Can you work these out from the model? Positions are in its coordinate system, mm. Face numbers are marked on the shaded views. Give positions to 0.01 mm unless a question says otherwise; leave off trailing zeros. Order: outer loops, then holes, each group sorted by start corner. A loop starts at its lowest first (then second) coordinate and runs counter-clockwise, first axis right, second up. Notation, with made-up numbers: (70.25, -39.5) -> (85.25, -39.5) arc R20 ccw to (85.25, -14.5) -> close; hole circle Ø4 at (-2, 41). An arc over 180 degrees is marked (long way). Answer as a JSON object with one key per item and string values.
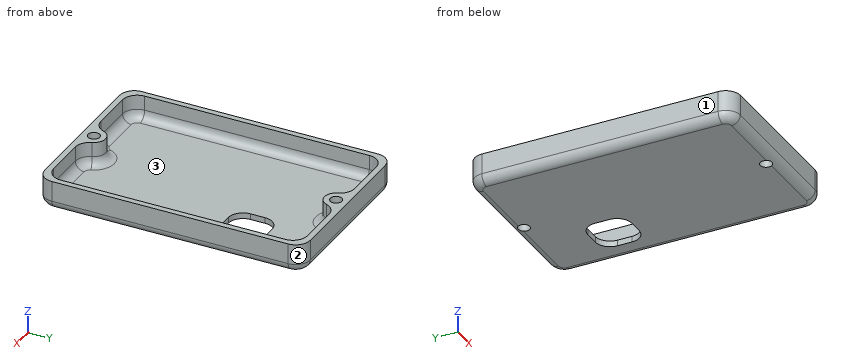
```python
from build123d import *

# Parameters (mm, degrees)
F3_W          = 60
F3_H          = 91
F4_DEPTH      = 10
F5_W          = 56
F5_H          = 87
F6_DEPTH      = 8
F7_R          = 4
F8_DEPTH      = 10
F9_R          = 2
F10_DEPTH     = 10.001
F11_R         = 5
F12_R         = 5
F13_T1_DEPTH  = 77
F13_T3_DEPTH  = 14.5147186258
F13_T5_DEPTH  = 14.5147186258
F13_T8_ANGLE  = 90
F13_T10_ANGLE = 70.5287793655
F13_T12_ANGLE = 141.057558731
F13_T14_ANGLE = 90
F13_T16_ANGLE = 70.5287793655
F13_T18_ANGLE = 70.5287793655
F13_T20_ANGLE = 90
F13_T22_ANGLE = 141.057558731
F13_T24_ANGLE = 70.5287793655
F13_T26_ANGLE = 90
F13_T27_DEPTH = 81
F13_T29_DEPTH = 50
F13_T32_ANGLE = 90
F13_T34_ANGLE = 90
F13_T36_ANGLE = 90
F13_T38_ANGLE = 90
F14_W         = 15
F14_H         = 15
F15_DEPTH     = 2.0010001
F16_R         = 5


# Not quite as in the source:
# - a fillet or chamfer that OpenCascade refuses, or shapes differently, is made with other operations: its cross-section is extruded or revolved along the edge and cut away or added


with BuildPart() as f4:
    # F3 (on Top) → F4 (new body)
    with BuildSketch(Plane.XY):
        Rectangle(F3_W, F3_H)
    extrude(amount=F4_DEPTH)

    # F5 (on face) → F6 (cut)
    with BuildSketch(Plane.XY.offset(10)):
        Rectangle(F5_W, F5_H)
    extrude(amount=-F6_DEPTH, mode=Mode.SUBTRACT)

    # F7 (on face) → F8 (join)
    with BuildSketch(Plane(origin=(0, 0, 0), x_dir=(1, 0, 0), z_dir=(0, 0, -1))):
        with Locations((0, -41.5)):
            Circle(F7_R)
        with Locations((0, 41.5)):
            Circle(F7_R)
    extrude(amount=-F8_DEPTH)

    # F9 (on face) → F10 (cut, through all)
    with BuildSketch(Plane(origin=(0, 0, 0), x_dir=(1, 0, 0), z_dir=(0, 0, -1))):
        with Locations((0, -41.5)):
            Circle(F9_R)
        with Locations((0, 41.5)):
            Circle(F9_R)
    extrude(amount=-F10_DEPTH, mode=Mode.SUBTRACT)

    # F11
    f11_edges = [f4.edges().sort_by_distance(p)[0] for p in [
        (3.464102, 43.5, 6),
        (-3.464102, 43.5, 6),
        (-3.464102, -43.5, 6),
        (3.464102, -43.5, 6),
    ]]
    fillet(f11_edges, radius=F11_R)

    # F12
    f12_edges = [f4.edges().sort_by_distance(p)[0] for p in [
        (30, -45.5, 5),
        (-30, -45.5, 5),
        (30, 45.5, 5),
        (-30, 45.5, 5),
        (28, -43.5, 6),
        (-28, -43.5, 6),
        (-28, 43.5, 6),
        (28, 43.5, 6),
    ]]
    fillet(f12_edges, radius=F12_R)

    # F13: fillet of radius 3 on 24 edges, made by hand

    # F13_s2 → F13_t1 (join)
    with BuildSketch(Plane.XZ.offset(-38.5)):
        with BuildLine():
            ThreePointArc((-28, 5), (-27.1213203436, 2.8786796564), (-25, 2))
            Line((-25, 2), (-28, 2))
            Line((-28, 2), (-28, 5))
        make_face()
        with BuildLine():
            ThreePointArc((28, 5), (27.1213203436, 2.8786796564), (25, 2))
            Line((25, 2), (28, 2))
            Line((28, 2), (28, 5))
        make_face()
    extrude(amount=F13_T1_DEPTH)

    # F13_s4 → F13_t3 (join)
    with BuildSketch(Plane.YZ.offset(8.4852813742)):
        with BuildLine():
            ThreePointArc((-43.5, 5), (-42.6213203436, 2.8786796564), (-40.5, 2))
            Line((-40.5, 2), (-43.5, 2))
            Line((-43.5, 2), (-43.5, 5))
        make_face()
        with BuildLine():
            ThreePointArc((43.5, 5), (42.6213203436, 2.8786796564), (40.5, 2))
            Line((40.5, 2), (43.5, 2))
            Line((43.5, 2), (43.5, 5))
        make_face()
    extrude(amount=F13_T3_DEPTH)

    # F13_s6 → F13_t5 (join)
    with BuildSketch(Plane.YZ.offset(-23)):
        with BuildLine():
            ThreePointArc((-43.5, 5), (-42.6213203436, 2.8786796564), (-40.5, 2))
            Line((-40.5, 2), (-43.5, 2))
            Line((-43.5, 2), (-43.5, 5))
        make_face()
        with BuildLine():
            ThreePointArc((43.5, 5), (42.6213203436, 2.8786796564), (40.5, 2))
            Line((40.5, 2), (43.5, 2))
            Line((43.5, 2), (43.5, 5))
        make_face()
    extrude(amount=F13_T5_DEPTH)

    # F13_s7 → F13_t8 (revolve)
    with BuildSketch(Plane.YZ.offset(23)):
        with BuildLine():
            ThreePointArc((-43.5, 5), (-42.6213203436, 2.8786796564), (-40.5, 2))
            Line((-40.5, 2), (-43.5, 2))
            Line((-43.5, 2), (-43.5, 5))
        make_face()
    revolve(axis=Axis((23, -38.5, 2), (0, 0, 1)), revolution_arc=F13_T8_ANGLE)

    # F13_s9 → F13_t10 (revolve)
    with BuildSketch(Plane.YZ.offset(8.4852813742)):
        with BuildLine():
            ThreePointArc((-43.5, 5), (-42.6213203436, 2.8786796564), (-40.5, 2))
            Line((-40.5, 2), (-43.5, 2))
            Line((-43.5, 2), (-43.5, 5))
        make_face()
    revolve(axis=Axis((8.4852813742, -38.5, 2), (0, 0, -1)), revolution_arc=F13_T10_ANGLE)

    # F13_s11 → F13_t12 (revolve)
    with BuildSketch(Plane(origin=(-13.0421917419, -36.8888888889, 0), x_dir=(0, 0, 1), z_dir=(-0.3333333333, -0.9428090416, 0))):
        with BuildLine():
            ThreePointArc((5, -9.8333333333), (2.8786796564, -8.9546536769), (2, -6.8333333333))
            Line((2, -6.8333333333), (2, -9.8333333333))
            Line((2, -9.8333333333), (5, -9.8333333333))
        make_face()
    revolve(axis=Axis((0, -41.5, 2), (0, 0, -1)), revolution_arc=F13_T12_ANGLE)

    # F13_s13 → F13_t14 (revolve)
    with BuildSketch(Plane.XZ.offset(-38.5)):
        with BuildLine():
            ThreePointArc((28, 5), (27.1213203436, 2.8786796564), (25, 2))
            Line((25, 2), (28, 2))
            Line((28, 2), (28, 5))
        make_face()
    revolve(axis=Axis((23, 38.5, 2), (0, 0, 1)), revolution_arc=F13_T14_ANGLE)

    # F13_s15 → F13_t16 (revolve)
    with BuildSketch(Plane(origin=(-13.0421917419, -36.8888888889, 0), x_dir=(0, 0, 1), z_dir=(0.3333333333, 0.9428090416, 0))):
        with BuildLine():
            ThreePointArc((5, 9.8333333333), (2.8786796564, 8.9546536769), (2, 6.8333333333))
            Line((2, 6.8333333333), (2, 9.8333333333))
            Line((2, 9.8333333333), (5, 9.8333333333))
        make_face()
    revolve(axis=Axis((-8.4852813742, -38.5, 2), (0, 0, -1)), revolution_arc=F13_T16_ANGLE)

    # F13_s17 → F13_t18 (revolve)
    with BuildSketch(Plane.YZ.offset(8.4852813742)):
        with BuildLine():
            ThreePointArc((43.5, 5), (42.6213203436, 2.8786796564), (40.5, 2))
            Line((40.5, 2), (43.5, 2))
            Line((43.5, 2), (43.5, 5))
        make_face()
    revolve(axis=Axis((8.4852813742, 38.5, 2), (0, 0, 1)), revolution_arc=F13_T18_ANGLE)

    # F13_s19 → F13_t20 (revolve)
    with BuildSketch(Plane.YZ.offset(-23)):
        with BuildLine():
            ThreePointArc((-43.5, 5), (-42.6213203436, 2.8786796564), (-40.5, 2))
            Line((-40.5, 2), (-43.5, 2))
            Line((-43.5, 2), (-43.5, 5))
        make_face()
    revolve(axis=Axis((-23, -38.5, 2), (0, 0, -1)), revolution_arc=F13_T20_ANGLE)

    # F13_s21 → F13_t22 (revolve)
    with BuildSketch(Plane(origin=(13.0421917419, 36.8888888889, 0), x_dir=(0, 0, 1), z_dir=(0.3333333333, 0.9428090416, 0))):
        with BuildLine():
            ThreePointArc((5, -9.8333333333), (2.8786796564, -8.9546536769), (2, -6.8333333333))
            Line((2, -6.8333333333), (2, -9.8333333333))
            Line((2, -9.8333333333), (5, -9.8333333333))
        make_face()
    revolve(axis=Axis((0, 41.5, 2), (0, 0, -1)), revolution_arc=F13_T22_ANGLE)

    # F13_s23 → F13_t24 (revolve)
    with BuildSketch(Plane(origin=(-13.0421917419, 36.8888888889, 0), x_dir=(0, 0, 1), z_dir=(0.3333333333, -0.9428090416, 0))):
        with BuildLine():
            ThreePointArc((5, -9.8333333333), (2.8786796564, -8.9546536769), (2, -6.8333333333))
            Line((2, -6.8333333333), (2, -9.8333333333))
            Line((2, -9.8333333333), (5, -9.8333333333))
        make_face()
    revolve(axis=Axis((-8.4852813742, 38.5, 2), (0, 0, 1)), revolution_arc=F13_T24_ANGLE)

    # F13_s25 → F13_t26 (revolve)
    with BuildSketch(Plane.XZ.offset(-38.5)):
        with BuildLine():
            ThreePointArc((-28, 5), (-27.1213203436, 2.8786796564), (-25, 2))
            Line((-25, 2), (-28, 2))
            Line((-28, 2), (-28, 5))
        make_face()
    revolve(axis=Axis((-23, 38.5, 2), (0, 0, -1)), revolution_arc=F13_T26_ANGLE)

    # F13_s28 → F13_t27 (cut)
    with BuildSketch(Plane.XZ.offset(-40.5)):
        with BuildLine():
            ThreePointArc((30, 3), (29.1213203436, 0.8786796564), (27, 0))
            Line((27, 0), (30, 0))
            Line((30, 0), (30, 3))
        make_face()
        with BuildLine():
            ThreePointArc((-30, 3), (-29.1213203436, 0.8786796564), (-27, 0))
            Line((-27, 0), (-30, 0))
            Line((-30, 0), (-30, 3))
        make_face()
    extrude(amount=F13_T27_DEPTH, mode=Mode.SUBTRACT)

    # F13_s30 → F13_t29 (cut)
    with BuildSketch(Plane.YZ.offset(-25)):
        with BuildLine():
            ThreePointArc((-45.5, 3), (-44.6213203436, 0.8786796564), (-42.5, 0))
            Line((-42.5, 0), (-45.5, 0))
            Line((-45.5, 0), (-45.5, 3))
        make_face()
        with BuildLine():
            ThreePointArc((45.5, 3), (44.6213203436, 0.8786796564), (42.5, 0))
            Line((42.5, 0), (45.5, 0))
            Line((45.5, 0), (45.5, 3))
        make_face()
    extrude(amount=F13_T29_DEPTH, mode=Mode.SUBTRACT)

    # F13_s31 → F13_t32 (revolve, cut)
    with BuildSketch(Plane.YZ.offset(25)):
        with BuildLine():
            ThreePointArc((-45.5, 3), (-44.6213203436, 0.8786796564), (-42.5, 0))
            Line((-42.5, 0), (-45.5, 0))
            Line((-45.5, 0), (-45.5, 3))
        make_face()
    revolve(axis=Axis((25, -40.5, 0), (0, 0, 1)), revolution_arc=F13_T32_ANGLE, mode=Mode.SUBTRACT)

    # F13_s33 → F13_t34 (revolve, cut)
    with BuildSketch(Plane.YZ.offset(-25)):
        with BuildLine():
            ThreePointArc((-45.5, 3), (-44.6213203436, 0.8786796564), (-42.5, 0))
            Line((-42.5, 0), (-45.5, 0))
            Line((-45.5, 0), (-45.5, 3))
        make_face()
    revolve(axis=Axis((-25, -40.5, 0), (0, 0, -1)), revolution_arc=F13_T34_ANGLE, mode=Mode.SUBTRACT)

    # F13_s35 → F13_t36 (revolve, cut)
    with BuildSketch(Plane.XZ.offset(-40.5)):
        with BuildLine():
            ThreePointArc((30, 3), (29.1213203436, 0.8786796564), (27, 0))
            Line((27, 0), (30, 0))
            Line((30, 0), (30, 3))
        make_face()
    revolve(axis=Axis((25, 40.5, 0), (0, 0, 1)), revolution_arc=F13_T36_ANGLE, mode=Mode.SUBTRACT)

    # F13_s37 → F13_t38 (revolve, cut)
    with BuildSketch(Plane.XZ.offset(-40.5)):
        with BuildLine():
            ThreePointArc((-30, 3), (-29.1213203436, 0.8786796564), (-27, 0))
            Line((-27, 0), (-30, 0))
            Line((-30, 0), (-30, 3))
        make_face()
    revolve(axis=Axis((-25, 40.5, 0), (0, 0, -1)), revolution_arc=F13_T38_ANGLE, mode=Mode.SUBTRACT)

    # F14 (on face) → F15 (cut, through all)
    with BuildSketch(Plane.XY.offset(2)):
        with Locations((15, 18.5)):
            Rectangle(F14_W, F14_H)
    extrude(amount=-F15_DEPTH, mode=Mode.SUBTRACT)

    # F16
    f16_edges = [f4.edges().sort_by_distance(p)[0] for p in [
        (7.5, 26, 1),
        (22.5, 26, 1),
        (22.5, 11, 1),
        (7.5, 11, 1),
    ]]
    fillet(f16_edges, radius=F16_R)


solid = f4.part
```
1. Will these pins go through, and if not, where does the flat tip stop? pin 1 Ø1.6 at (x, z) = (14.5, 0.5) entering from +Y; pin 2 Ø5 at (y, z) = (-7, 2) entering from -X; pin 3 Ø0.6 at (y, z) = (19.5, 1) entering from +X; pin 4 Ø1 at (x, y) = (-12.5, 23.5) entering from +Z.
Worked answers:
{"pin 1": "y = 44.97", "pin 2": "x = -30", "pin 3": "x = 29.47", "pin 4": "z = 2"}
2. If we section it at A-A on x = 16.5: Please give me the cut outline in (y, z).
Worked answers:
{"outline": "(-45.5, 3) arc R3 ccw to (-42.5, 0) -> (11, 0) -> (11, 2) -> (-40.5, 2) arc R3 cw to (-43.5, 5) -> (-43.5, 10) -> (-45.5, 10) -> close; (26, 0) -> (42.5, 0) arc R3 ccw to (45.5, 3) -> (45.5, 10) -> (43.5, 10) -> (43.5, 5) arc R3 cw to (40.5, 2) -> (26, 2) -> close"}
3. If we section it at C-C on y = -27: Please give me the cut outline in (x, z), then the cut area to 3 significant figures.
Worked answers:
{"outline": "(-30, 3) arc R3 ccw to (-27, 0) -> (27, 0) arc R3 ccw to (30, 3) -> (30, 10) -> (28, 10) -> (28, 5) arc R3 cw to (25, 2) -> (-25, 2) arc R3 cw to (-28, 5) -> (-28, 10) -> (-30, 10) -> close", "area": "152 mm²"}
4. If we mould it in two halves opening along Y, with no side actions, what happens to the marked faces 1, 2 and 3? For each: +Y half, -Y half, draft (parallel to the pull), parting line (faces both ways), or undercut.
Worked answers:
{"face 1": "draft", "face 2": "+Y half", "face 3": "undercut"}
5. If we section it at D-D on x = 0: Please give me the cut outline in (y, z), then the cut area to 3 significant figures.
Worked answers:
{"outline": "(-45.5, 3) arc R3 ccw to (-43.5, 0.17) -> (-43.5, 10) -> (-45.5, 10) -> close; (-39.5, 0) -> (39.5, 0) -> (39.5, 10) -> (37.5, 10) -> (37.5, 5) arc R3 cw to (34.5, 2) -> (-34.5, 2) arc R3 cw to (-37.5, 5) -> (-37.5, 10) -> (-39.5, 10) -> close; (43.5, 0.17) arc R3 ccw to (45.5, 3) -> (45.5, 10) -> (43.5, 10) -> close", "area": "230 mm²"}
6. If we section it at B-B on z = 6: Please give me the cut outline in (x, y), then the cut area to 3 significant figures.
Worked answers:
{"outline": "(-30, -40.5) arc R5 ccw to (-25, -45.5) -> (25, -45.5) arc R5 ccw to (30, -40.5) -> (30, 40.5) arc R5 ccw to (25, 45.5) -> (-25, 45.5) arc R5 ccw to (-30, 40.5) -> close; hole (-28, -38.5) arc R5 ccw to (-23, -43.5) -> (-8.49, -43.5) arc R5 ccw to (-3.77, -40.17) arc R4 cw to (3.77, -40.17) arc R5 ccw to (8.49, -43.5) -> (23, -43.5) arc R5 ccw to (28, -38.5) -> (28, 38.5) arc R5 ccw to (23, 43.5) -> (8.49, 43.5) arc R5 ccw to (3.77, 40.17) arc R4 cw to (-3.77, 40.17) arc R5 ccw to (-8.49, 43.5) -> (-23, 43.5) arc R5 ccw to (-28, 38.5) -> close; hole circle Ø4 at (0, -41.5); hole circle Ø4 at (0, 41.5)", "area": "660 mm²"}
7. Please list where these lines run through material, in increasing order: L1, parallel to Y at x = 0, z = 5.5; L2, parallel to Y at x = -22, z = 8; L3, parallel to X at y = 41.5, z = 5.5.
Worked answers:
{"L1": "-45.5 to -43.5, -39.5 to -37.5, 37.5 to 39.5, 43.5 to 45.5", "L2": "-45.5 to -43.5, 43.5 to 45.5", "L3": "-29.9 to -27, -4.49 to -2, 2 to 4.49, 27 to 29.9"}
